For this review, take the finished solid that the model builds, in its own axes (mm). A direction names the side the tool comes from. Give positions to 0.01 mm unless a question says otherwise; leave off trailing zeros. Order: outer loops, then holes, each group sorted by start corner. A loop starts at its lowest first (then second) coordinate and runs counter-clockwise, first axis right, second up.
from build123d import *

# Parameters (mm, degrees)
SKETCH1_R           = 52.5
SKETCH1_R_2         = 37.5
BOSS_EXTRUDE1_DEPTH = 2
SKETCH2_R           = 52.5
SKETCH2_R_2         = 42.75
BOSS_EXTRUDE2_DEPTH = 1.5
SKETCH3_R           = 1.65
CUT_EXTRUDE1_DEPTH  = 75.328662036
CIRPATTERN1_COUNT   = 12


with BuildPart() as part:
    # Sketch1 → Boss-Extrude1 (new body)
    with BuildSketch(Plane(origin=(0, 0, 0), x_dir=(1, 0, 0), z_dir=(0, 1, 0))):
        with Locations(Location((0, 0, 0), (0, 0, 270))):
            Circle(SKETCH1_R)
        with Locations(Location((0, 0, 0), (0, 0, 270))):
            Circle(SKETCH1_R_2, mode=Mode.SUBTRACT)
    extrude(amount=BOSS_EXTRUDE1_DEPTH)

    # Sketch2 → Boss-Extrude2 (add)
    with BuildSketch(Plane(origin=(0, 2, 0), x_dir=(1, 0, 0), z_dir=(0, 1, 0))):
        with Locations(Location((0, 0, 0), (0, 0, 270))):
            Circle(SKETCH2_R)
        with Locations(Location((0, 0, 0), (0, 0, 270))):
            Circle(SKETCH2_R_2, mode=Mode.SUBTRACT)
    extrude(amount=BOSS_EXTRUDE2_DEPTH)

    # Sketch3 → Cut-Extrude1 (cut, through all)
    with BuildSketch(Plane.XZ):
        with Locations(Location((47.5, 0, 0), (0, 0, 270))):
            Circle(SKETCH3_R)
    cut_extrude1 = extrude(amount=-CUT_EXTRUDE1_DEPTH, mode=Mode.SUBTRACT)

    # CirPattern1: Cut-Extrude1 ×12 about axis
    cirpattern1_axis = Axis((0, 0, 0), (0, 1, 0))
    for i in range(1, CIRPATTERN1_COUNT):
        add(cut_extrude1.rotate(cirpattern1_axis, i * 360 / CIRPATTERN1_COUNT), mode=Mode.SUBTRACT)


solid = part.part
1) Clearance check with flat-ended pins moving along their axes: pin 1 (1 mm diameter, centred on y = 2, z = -37, fed in from -X); pin 2 (1.5 mm diameter, centred on x = 16.5, y = 3, fed in from -Z); pin 3 (1 mm diameter, centred on x = -38, y = 3, fed in from +Z); pin 4 (2.5 mm diameter, centred on x = -23.75, z = -41.14, fed in from +Y). State where each tip first meets the part, or that it passes through.
Answer sheet:
pin 1: stops at x = -37.74
pin 2: stops at z = -50.08
pin 3: stops at z = 36.74
pin 4: passes through
2) We need section A-A on x = -35.5. Give the boundary of the cut face in (y, z), then the cut area to 3 significant figures.
Answer sheet:
outline: (0, -38.68) - (3.5, -38.68) - (3.5, -23.82) - (2, -23.82) - (2, -12.08) - (0, -12.08) - close; (0, 12.08) - (2, 12.08) - (2, 23.82) - (3.5, 23.82) - (3.5, 38.68) - (0, 38.68) - close
area: 151 mm2
3) We need section C-C on y = 1.45. Count the separate pieces of the cut face and the enclosed holes in it, then the cut area to 3 significant figures.
Answer sheet:
separate pieces: 1
enclosed holes: 13
area: 4,140 mm2
4) Tool access review of faces 4 (the face through (42.386, 2.74, -5.565)), 5 (the face through (23.254, 1.726, -39.562)): name each direction out of +Z, -Z, +X, -X, +Y, -Y from which nothing blocks a thin tool from reaching the whole face with its end or side.
Answer sheet:
face 4: +Y
face 5: +Y, -Y
5) We need section D-D on x = 23.75. Give the boundary of the cut face in (y, z), then the cut area to 3 significant figures.
Answer sheet:
outline: (0, -46.82) - (3.5, -46.82) - (3.5, -42.79) - (0, -42.79) - close; (0, -39.49) - (3.5, -39.49) - (3.5, -35.55) - (2, -35.55) - (2, -29.02) - (0, -29.02) - close; (0, 29.02) - (2, 29.02) - (2, 35.55) - (3.5, 35.55) - (3.5, 39.49) - (0, 39.49) - close; (0, 42.79) - (3.5, 42.79) - (3.5, 46.82) - (0, 46.82) - close
area: 81.9 mm2
6) We need section B-B on z = 47.5. Give the boundary of the cut face in (x, y).
Answer sheet:
outline: (-22.36, 0) - (-1.65, 0) - (-1.65, 3.5) - (-22.36, 3.5) - close; (1.65, 0) - (22.36, 0) - (22.36, 3.5) - (1.65, 3.5) - close
7) Draft analysis for pull direction X (two halves, no side actions). For faces 1 (the face through (-0.89, 1.73, -48.89)), 2 (the face through (15.77, 1.726, 50.076)), 3 (the face through (-4, 3.5, -43)), state which applies: +X half, -X half, draft (parallel to the pull), parting line (faces both ways), or undercut.
Answer sheet:
face 1: undercut
face 2: parting line
face 3: draft
8) To check wall thickness, follow line 1 (X direction, y = 1.3, z = -24); line 2 (Y direction, x = 34.5, z = -21.5); line 3 (X direction, y = 0.95, z = -5). State the ranges of each line that lie inside material, in increasing order.
Answer sheet:
line 1: x = -46.69 to -42.77, -39.51 to -28.81, 28.81 to 39.51, 42.77 to 46.69
line 2: y = 0 to 2
line 3: x = -52.26 to -37.17, 37.17 to 52.26
